from build123d import *

# Parameters (mm, degrees)
PAD_DEPTH    = 6.5
PAD001_DEPTH = 4
PAD002_DEPTH = 10


with BuildPart() as cuerpo:
    # Sketch → Pad (new body)
    with BuildSketch(Plane.XY):
        Polygon((0, 7.505553), (-6.5, 3.752777), (-6.5, -3.752777), (0, -7.505553), (6.5, -3.752777), (6.5, 3.752777), align=None)
    extrude(amount=PAD_DEPTH)

    # Sketch001 (on Face8 of Pad) → Pad001 (join)
    with BuildSketch(Plane.XY.offset(6.5)):
        Polygon((0, 5.773503), (-5, 2.886751), (-5, -2.886751), (0, -5.773503), (5, -2.886751), (5, 2.886751), align=None)
    extrude(amount=PAD001_DEPTH)


with BuildPart() as cut:
    # Sketch002 → Pad002 (new body)
    with BuildSketch(Plane.XY):
        Polygon((0, 9.814955), (-8.5, 4.907477), (-8.5, -4.907477), (0, -9.814955), (8.5, -4.907477), (8.5, 4.907477), align=None)
    extrude(amount=PAD002_DEPTH)

    # Cut: cut Cuerpo
    add(cuerpo.part, mode=Mode.SUBTRACT)


solid = cut.part
Part model, mm, in its own coordinate system. A direction names the side the tool comes from. Coordinates: 2 decimals unless noted, no trailing zeros. Write each loop counter-clockwise with the first axis right and the second up, starting at its lowest first coordinate (ties: lowest second). Pieces come first, ordered by that corner, then holes. Notation, with made-up numbers: (74.5, 73.5) - (81.5, 73.5) arc R19 ccw to (81.5, 98.5) - close; hole circle Ø10 at (-8.5, 53.5). An arc over 180 degrees is marked (long way). Put each result on its own line as item: value.
1. Band-saw the part on D-D (z = 5.75). Write the cut outline in (x, y), then the cut area to 3 significant figures.
Final values:
outline: (-8.5, -4.91) - (0, -9.81) - (8.5, -4.91) - (8.5, 4.91) - (0, 9.81) - (-8.5, 4.91) - close; hole (-6.5, -3.75) - (0, -7.51) - (6.5, -3.75) - (6.5, 3.75) - (0, 7.51) - (-6.5, 3.75) - close
area: 104 mm²
2. Probe line 1 along X through (y, z) = (1.75, 8.75); line 2 along X through (y, z) = (3.5, 3.5); line 3 along Z through (x, y) = (-4.75, 3.25). List the from-to ranges inside material, lowest first. Write a range as [from, to].
Final values:
line 1: x = [-8.5, -5], [5, 8.5]
line 2: x = [-8.5, -6.5], [6.5, 8.5]
line 3: z = [6.5, 10]
3. Band-saw the part on A-A (y = 2.25). Write the cut outline in (x, z).
Final values:
outline: (-8.5, 0) - (-6.5, 0) - (-6.5, 6.5) - (-5, 6.5) - (-5, 10) - (-8.5, 10) - close; (5, 6.5) - (6.5, 6.5) - (6.5, 0) - (8.5, 0) - (8.5, 10) - (5, 10) - close
4. 3-axis set-ups, long thin cutter, end or side, ignore diameter. For faces 4 (the flat face through (-4.19, 7.396, 4.93)), 5 (the flat face through (-3.2, 5.66, 3.2)), 6 (the flat face through (5, 0, 8)): which of +Z, -Z, +X, -X, +Y, -Y reach the whole face in a straight line?
Final values:
face 4: +Z, -Z, -X, +Y
face 5: -Z
face 6: +Z, -Z
5. Band-saw the part on C-C (x = -3.5). Write the cut outline in (y, z), then the cut area to 3 significant figures.
Final values:
outline: (-7.79, 0) - (-5.48, 0) - (-5.48, 6.5) - (-3.75, 6.5) - (-3.75, 10) - (-7.79, 10) - close; (3.75, 6.5) - (5.48, 6.5) - (5.48, 0) - (7.79, 0) - (7.79, 10) - (3.75, 10) - close
area: 58.3 mm²
6. Band-saw the part on B-B (z = 7.5). Write the cut outline in (x, y), then the cut area to 3 significant figures.
Final values:
outline: (-8.5, -4.91) - (0, -9.81) - (8.5, -4.91) - (8.5, 4.91) - (0, 9.81) - (-8.5, 4.91) - close; hole (-5, -2.89) - (0, -5.77) - (5, -2.89) - (5, 2.89) - (0, 5.77) - (-5, 2.89) - close
area: 164 mm²
7. Flat gauge pins, fed straight in: pin 1 Ø5 at (x, z) = (4, 3.5) entering from +Y; pin 2 Ø3 at (x, z) = (6, 6) entering from +Y; pin 3 Ø10 at (x, y) = (1, -0.5) entering from -Z. Where does each tip first touch, or does it go through?
Final values:
pin 1: stops at y = 8.95
pin 2: stops at y = 7.22
pin 3: stops at z = 6.5
8. Two-plate mould, pull along Y, no slides. Class faces 1 (the flat face through (8.5, 0, 5)), 2 (the flat face through (4.19, -7.396, 4.93)), 3 (the flat face through (-3.3, -5.6, 3.2)): +Y half, -Y half, draft (parallel to the pull), parting line (faces both ways), or undercut.
Final values:
face 1: draft
face 2: -Y half
face 3: undercut
